Model file for the job. Use its own axes, mm. A direction names the side the tool comes from. Give positions to 0.01 mm unless a question says otherwise; leave off trailing zeros. Loops run counter-clockwise (first coordinate to the right, second up) from the corner with the lowest first, then second, coordinate; pieces in that order, holes last. Notation, with made-up numbers: (-11, 45) - (15, 45) arc R24 cw to (15, 78) - close; hole circle Ø2 at (-32, 8). An arc over 180 degrees is marked (long way). Use a Markdown table: item, result.
Autodesk Inventor part; units mm, degrees
ref_plane "YZ Plane" through (0, 0, 0) normal (1, 0, 0) x (0, 1, 0)
ref_plane "XZ Plane" through (0, 0, 0) normal (0, 1, 0) x (-1, 0, 0)
ref_plane "XY Plane" through (0, 0, 0) normal (0, 0, 1) x (1, 0, 0)
sketch "スケッチ1" plane through (0, 0, 0) normal (0, 0, 1) x (1, 0, 0)
  line L0 (0, 0) -> (90, 0)
  line L1 (90, 0) -> (90, 90)
  line L2 (90, 90) -> (0, 90)
  line L3 (0, 90) -> (0, 0)
  line L4 (0, 10) -> (90, 10) construction
  circle A0 centre (10, 10) radius 2.5
  circle A1 centre (80, 10) radius 2.5
  circle A2 centre (18.5, 81.5) radius 1.6
  circle A3 centre (18.5, 28.5) radius 1.6
  circle A4 centre (71.5, 81.5) radius 1.6
  circle A5 centre (71.5, 28.5) radius 1.6
  line L5 (18.5, 81.5) -> (18.5, 28.5) construction
  line L6 (18.5, 28.5) -> (71.5, 28.5) construction
  line L7 (71.5, 28.5) -> (71.5, 81.5) construction
  line L8 (71.5, 81.5) -> (18.5, 81.5) construction
  line L9 (45, 90) -> (45, 0) construction
  line L10 (0, 55) -> (90, 55) construction
  line L11 (49.95, 50.05) -> (40.05, 50.05) construction
  line L12 (40.05, 50.05) -> (40.05, 59.95) construction
  line L13 (40.05, 59.95) -> (49.95, 59.95) construction
  line L14 (49.95, 59.95) -> (49.95, 50.05) construction
  line L15 (49.95, 50.05) -> (40.05, 59.95) construction
  line L16 (40.05, 50.05) -> (49.95, 59.95) construction
  circle A6 centre (49.95, 59.95) radius 1.6
  circle A7 centre (40.05, 59.95) radius 1.6
  circle A8 centre (49.95, 50.05) radius 1.6
  circle A9 centre (40.05, 50.05) radius 1.6
  circle A10 centre (45, 55) radius 1.6
  dimension "d0" = 5
  dimension "d1" = 10
  dimension "d2" = 10
  dimension "d3" = 10
  dimension "d4" = 90
  dimension "d5" = 90
  dimension "d12" = 3.2
  dimension "d21" = 53
  dimension "d23" = 53
  dimension "d33" = 55
  dimension "d34" = 3.2
  dimension "d35" = 9.9
  dimension "d36" = 9.9
extrude "押し出し1" add sketch "スケッチ1" along normal blind 3
sketch "スケッチ2" plane through (0, 0, 3) normal (0, 0, 1) x (1, 0, 0)
  line L0 (90, 90) -> (0, 90) construction
  line L1 (45, 90) -> (45, 0) construction
  line L2 (45, 77.4767) -> (82.4767, 40) construction
  line L3 (82.4767, 40) -> (45, 2.5233) construction
  line L4 (45, 2.5233) -> (7.5233, 40) construction
  line L5 (7.5233, 40) -> (45, 77.4767) construction
  line L6 (45, 77.4767) -> (45, 2.5233) construction
  line L7 (82.4767, 40) -> (7.5233, 40) construction
  line L8 (0, 0) -> (90, 0) construction
  circle A0 centre (82.4767, 40) radius 1.5
  circle A1 centre (45, 77.4767) radius 1.5
  circle A2 centre (45, 2.5233) radius 1.5 construction
  circle A3 centre (7.5233, 40) radius 1.5
  point P0 (45, 40)
  dimension "d27" = 53
  dimension "d28" = 90
  dimension "d29" = 40
  dimension "d30" = 3
extrude "押し出し2" cut sketch "スケッチ2" against normal up to next
fillet "フィレット2" radius 5 4 edges at (90, 90, 1.5) (0, 90, 1.5) (90, 0, 1.5) (0, 0, 1.5)
sketch "スケッチ3" plane through (0, 0, 0) normal (0, 0, -1) x (-1, 0, 0)
  line L0 (-70, 65.05) -> (-20, 65.05)
  line L1 (-20, 65.05) -> (-20, 44.95)
  line L2 (-20, 44.95) -> (-70, 44.95)
  line L3 (-70, 44.95) -> (-70, 65.05)
  circle A0 centre (-45, 55) radius 1.6
  line L4 (-70, 65.05) -> (-20, 44.95) construction
  line L5 (-20, 65.05) -> (-70, 44.95) construction
  point P0 (0, 0)
  dimension "d38" = 20.1
  dimension "d39" = 50
extrude "押し出し3" cut sketch "スケッチ3" against normal blind 1
fillet "フィレット3" radius 2 4 edges at (70, 65.05, 0.5) (20, 65.05, 0.5) (20, 44.95, 0.5) (70, 44.95, 0.5)
properties part number "LRFマウント"
(1) Slice it at A-A, the plane y = 40. Write the cut outline in (x, z), plus the area to 3 significant figures.
Computed:
| item | result |
|---|---|
| outline | (0, 0) - (6.02, 0) - (6.02, 3) - (0, 3) - close; (9.02, 0) - (80.98, 0) - (80.98, 3) - (9.02, 3) - close; (83.98, 0) - (90, 0) - (90, 3) - (83.98, 3) - close |
| area | 252 mm² |
(2) Mould opens along X. For faces 1 (the cylindrical face through (73.026, 28.019, 1.479)), 2 (the flat face through (46, 90, 1)), 3 (the cylindrical face through (2, 89, 2)), 4 (the cylindrical face through (48.77, 58.87, 1.99)) say: pulls with the +X half, pulls with the -X half, needs draft (parallel to the pull), parting line crosses it, or undercut.
Computed:
| item | result |
|---|---|
| face 1 | undercut |
| face 2 | needs draft |
| face 3 | pulls with the -X half |
| face 4 | undercut |
(3) Pin check, flat tips, straight feed: P1, Ø5, axis at x = 7.52, y = 40, coming from the -Z side; P2, Ø16, axis at x = 38, y = 56, coming from the -Z side. Stop position of each tip, or through.
Computed:
| item | result |
|---|---|
| P1 | z = 0 |
| P2 | z = 1 |
(4) 3-axis set-ups, long thin cutter, end or side, ignore diameter. For faces 5 (the cylindrical face through (69.4, 45.52, 0.51)), 6 (the cylindrical face through (41.576, 49.569, 1.986)): which of +Z, -Z, +X, -X, +Y, -Y reach the whole face in a straight line?
Computed:
| item | result |
|---|---|
| face 5 | -Z |
| face 6 | +Z, -Z |
(5) Drill centre lines: probe 1 along Y at (x, z) = (45, 1.85); probe 2 along Y at (x, z) = (71.5, 1.85); probe 3 along X at (y, z) = (50.05, 2.05). Where is each one in solid material? Low to high. Write a range as [from, to].
Computed:
| item | result |
|---|---|
| probe 1 | [0, 53.4], [56.6, 75.98], [78.98, 90] |
| probe 2 | [0, 26.9], [30.1, 79.9], [83.1, 90] |
| probe 3 | [0, 38.45], [41.65, 48.35], [51.55, 90] |
(6) Slice it at B-B, the plane x = 49.95. Write the cut outline in (y, z), plus the area to 3 significant figures.
Computed:
| item | result |
|---|---|
| outline | (0, 0) - (44.95, 0) - (44.95, 1) - (48.45, 1) - (48.45, 3) - (0, 3) - close; (51.65, 1) - (58.35, 1) - (58.35, 3) - (51.65, 3) - close; (61.55, 1) - (65.05, 1) - (65.05, 0) - (90, 0) - (90, 3) - (61.55, 3) - close |
| area | 237 mm² |
(7) Slice it at C-C, the plane x = 35. Write the cut outline in (y, z).
Computed:
| item | result |
|---|---|
| outline | (0, 0) - (44.95, 0) - (44.95, 1) - (65.05, 1) - (65.05, 0) - (90, 0) - (90, 3) - (0, 3) - close |
(8) Slice it at D-D, the plane y = 55. Write the cut outline in (x, z), plus the area to 3 significant figures.
Computed:
| item | result |
|---|---|
| outline | (0, 0) - (20, 0) - (20, 1) - (43.4, 1) - (43.4, 3) - (0, 3) - close; (46.6, 1) - (70, 1) - (70, 0) - (90, 0) - (90, 3) - (46.6, 3) - close |
| area | 214 mm² |
